from build123d import *

# Parameters (mm, degrees)
F0_R     = 3.75
F1_DEPTH = 25


with BuildPart() as f1:
    # F0 (on Top) → F1 (new body)
    with BuildSketch(Plane.XY):
        with BuildLine():
            ThreePointArc((-7.75, 22.3), (-11.152254, 18.897746), (-14.554509, 22.3))
            ThreePointArc((-14.554509, 22.3), (-12.821388, 26.540759), (-14, 30.967793))
            Line((-14, 30.967793), (-14, 34.967793))
            Line((-14, 34.967793), (-16, 34.967793))
            Line((-16, 34.967793), (-16, 29.467793))
            ThreePointArc((-16, 29.467793), (-15.895818, 24.709653), (-20, 22.3))
            ThreePointArc((-20, 22.3), (-24.104182, 24.709653), (-24, 29.467793))
            Line((-24, 29.467793), (-24, 34.967793))
            Line((-24, 34.967793), (-26, 34.967793))
            Line((-26, 34.967793), (-26, 30.967793))
            ThreePointArc((-26, 30.967793), (-27.178612, 26.540759), (-25.445491, 22.3))
            Line((-25.445491, 22.3), (-45.445491, 22.3))
            Line((-45.445491, 22.3), (-45.445491, -24))
            Line((-45.445491, -24), (-14, -24))
            ThreePointArc((-14, -24), (-9.899495, -14.100505), (0, -10))
            ThreePointArc((0, -10), (9.899495, -14.100505), (14, -24))
            Line((14, -24), (45.445491, -24))
            Line((45.445491, -24), (45.445491, 22.3))
            Line((45.445491, 22.3), (25.445491, 22.3))
            ThreePointArc((25.445491, 22.3), (27.178612, 26.540759), (26, 30.967793))
            Line((26, 30.967793), (26, 34.967793))
            Line((26, 34.967793), (24, 34.967793))
            Line((24, 34.967793), (24, 29.467793))
            ThreePointArc((24, 29.467793), (24.104182, 24.709653), (20, 22.3))
            ThreePointArc((20, 22.3), (15.895818, 24.709653), (16, 29.467793))
            Line((16, 29.467793), (16, 34.967793))
            Line((16, 34.967793), (14, 34.967793))
            Line((14, 34.967793), (14, 30.967793))
            ThreePointArc((14, 30.967793), (12.821388, 26.540759), (14.554509, 22.3))
            ThreePointArc((14.554509, 22.3), (11.152254, 18.897746), (7.75, 22.3))
            Line((7.75, 22.3), (7.75, 40))
            ThreePointArc((7.75, 40), (5.480078, 45.480078), (0, 47.75))
            ThreePointArc((0, 47.75), (-5.480078, 45.480078), (-7.75, 40))
            Line((-7.75, 40), (-7.75, 22.3))
        make_face()
        with Locations((0, 40)):
            Circle(F0_R, mode=Mode.SUBTRACT)
    extrude(amount=F1_DEPTH)


solid = f1.part
Source: CAD feature listing. Evaluate the final solid. Frame: model axes, mm. A direction names the side the tool comes from. Round coordinates to 2 decimals unless told otherwise and drop trailing zeros. Order: outer loops, then holes, each group sorted by start corner. A loop starts at its lowest first (then second) coordinate and runs counter-clockwise, first axis right, second up. Notation, with made-up numbers: (50.25, 55.25) - (100.25, 55.25) arc R12 cw to (100.25, 78.25) - close; hole circle Ø5 at (-39.75, -34.5). An arc over 180 degrees is marked (long way). Use a Markdown table: item, result. Add a question column.
1. Mould query, pull axis Y, two halves, no side actions, for faces 1 (the flat face through (-26, 33, 12)), 2 (the cylindrical face through (-11.1, 18.9, 12.3)), 3 (the flat face through (-30, -24, 12)), 4 (the cylindrical face through (-27.182, 26.606, 12.325)). Classes: +Y half, -Y half, draft (parallel to the pull), parting line (faces both ways), or undercut.
2. Section query D-D (x = -17). Return the cut outline in (y, z), then the cut area to 3 significant figures.
3. Line query: probe 1 along X at (y, z) = (31.5, 16.5); probe 2 along X at (y, z) = (27, 2.75); probe 3 along Y at (x, z) = (-37.5, 17.5). Output: solid intervals per line, ascending.
4. First-contact query: pin 1 (1.2 mm diameter, centred on y = 33, z = 8.5, fed in from -X); pin 2 (4.5 mm diameter, centred on y = 32.5, z = 14, fed in from -X); pin 3 (1 mm diameter, centred on x = 25.5, z = 10, fed in from +Y); pin 4 (7 mm diameter, centred on x = 0, y = 40, fed in from -Z). Flat tips, straight axial feed; report the tip coordinate or a pass-through.
5. Section query A-A (y = -14). Return the cut outline in (x, z).
6. Section query C-C (x = 34). Return the cut outline in (y, z).
7. Section query B-B (y = 21). Return the cut outline in (x, z), then the cut area to 3 significant figures.
8. Set-up query: faces 5 (the flat face through (-24, 32, 12)), 6 (the cylindrical face through (11.2, 18.9, 12.3)), 7 (the flat face through (15, 34.968, 12)), 8 (the flat face through (-25, 34.968, 12)). Return all of +Z, -Z, +X, -X, +Y, -Y with unobstructed straight access to the full face (end or side cutting, diameter ignored); none if empty.
Derived:
| question | item | result |
|---|---|---|
| 1 | face 1 | draft |
| 1 | face 2 | undercut |
| 1 | face 3 | -Y half |
| 1 | face 4 | undercut |
| 2 | outline | (-24, 0) - (23.38, 0) - (23.38, 25) - (-24, 25) - close |
| 2 | area | 1,180 mm2 |
| 3 | probe 1 | -26 to -24, -16 to -14, -7.75 to 7.75, 14 to 16, 24 to 26 |
| 3 | probe 2 | -27.19 to -24.7, -15.3 to -12.81, -7.75 to 7.75, 12.81 to 15.3, 24.7 to 27.19 |
| 3 | probe 3 | -24 to 22.3 |
| 4 | pin 1 | x = -26 |
| 4 | pin 2 | x = -26.42 |
| 4 | pin 3 | y = 34.97 |
| 4 | pin 4 | through |
| 5 | outline | (-45.45, 0) - (-9.8, 0) - (-9.8, 25) - (-45.45, 25) - close; (9.8, 0) - (45.45, 0) - (45.45, 25) - (9.8, 25) - close |
| 6 | outline | (-24, 0) - (22.3, 0) - (22.3, 25) - (-24, 25) - close |
| 7 | outline | (-45.45, 0) - (-14.3, 0) - (-14.3, 25) - (-45.45, 25) - close; (-8.01, 0) - (8.01, 0) - (8.01, 25) - (-8.01, 25) - close; (14.3, 0) - (45.45, 0) - (45.45, 25) - (14.3, 25) - close |
| 7 | area | 1,960 mm2 |
| 8 | face 5 | +Z, -Z, +Y |
| 8 | face 6 | +Z, -Z |
| 8 | face 7 | +Z, -Z, +X, +Y |
| 8 | face 8 | +Z, -Z, -X, +Y |
